```python
from build123d import *

# Parameters (mm, degrees)
SKETCH_1_W          = 113
SKETCH_1_H          = 50
SKETCH_1_R          = 1.6
SKETCH_1_R_2        = 8
SKETCH_1_R_3        = 6
EXTRUDE_1_DEPTH     = 4
SKETCH_2_R          = 1.5
SKETCH_2_R_2        = 1.6
SKETCH_2_R_3        = 2.1
CUT_EXTRUDE_1_DEPTH = 124.632519994


with BuildPart() as part:
    # ｽｹｯﾁ1 → ﾎﾞｽ - 押し出し1 (new body)
    with BuildSketch(Plane.XY):
        with Locations((56.5, 25)):
            Rectangle(SKETCH_1_W, SKETCH_1_H)
        with Locations((5, 45)):
            Circle(SKETCH_1_R, mode=Mode.SUBTRACT)
        with Locations((5, 5)):
            Circle(SKETCH_1_R, mode=Mode.SUBTRACT)
        with Locations((108, 45)):
            Circle(SKETCH_1_R, mode=Mode.SUBTRACT)
        with Locations((108, 5)):
            Circle(SKETCH_1_R, mode=Mode.SUBTRACT)
        with Locations((57.31, 25)):
            Circle(SKETCH_1_R_2, mode=Mode.SUBTRACT)
        with Locations((81.99, 25)):
            Circle(SKETCH_1_R_3, mode=Mode.SUBTRACT)
    extrude(amount=EXTRUDE_1_DEPTH)

    # ｽｹｯﾁ2 → ｶｯﾄ - 押し出し1 (cut, through all)
    with BuildSketch(Plane.XY.offset(4)):
        with Locations((90.39, 25)):
            Circle(SKETCH_2_R)
        with Locations((98.99, 46)):
            Circle(SKETCH_2_R_2)
        with Locations((98.99, 4)):
            Circle(SKETCH_2_R_2)
        with Locations((68.99, 4)):
            Circle(SKETCH_2_R_2)
        with Locations((68.99, 46)):
            Circle(SKETCH_2_R_2)
        with Locations((57.31, 39.5)):
            Circle(SKETCH_2_R_3)
        with Locations((57.31, 10.5)):
            Circle(SKETCH_2_R_3)
    extrude(amount=-CUT_EXTRUDE_1_DEPTH, mode=Mode.SUBTRACT)


solid = part.part
```
The listing builds one solid part. Answer for the finished solid, in the listing's coordinates (mm). Give positions to 0.01 mm unless a question says otherwise; leave off trailing zeros. Write each loop counter-clockwise with the first axis right and the second up, starting at its lowest first coordinate (ties: lowest second). Pieces come first, ordered by that corner, then holes. Notation, with made-up numbers: (21, 72) - (59, 72) arc R8 ccw to (59, 83) - close; hole circle Ø2 at (-8.5, 63). An arc over 180 degrees is marked (long way). Use one line per item in the form item = value. Start each with the question number.
1) Consider line 1 along Y through (x, z) = (98.99, 2.2); line 2 along Y through (x, z) = (57.31, 2.35); line 3 along X through (y, z) = (19.5, 2.4). Determine where each line is inside the solid, lowest interval first. Write a range as from..to.
2) Find section B-B on z = 1.65. Count the separate pieces of the cut face and the enclosed holes in it, plus the area to 3 significant figures.
3) The mould has two halves that part along Y. Classify faces 1 (the face through (56, 0, 2)), 2 (the face through (75.996, 25.264, 1.972)), 3 (the face through (56, 36, 0)): pulls with the +Y half, pulls with the -Y half, needs draft (parallel to the pull), parting line crosses it, or undercut.
4) Find section D-D on x = 81.99. Determine the outline of the cut face in (y, z), plus the area to 3 significant figures.
5) Find section C-C on y = 25. Determine the outline of the cut face in (x, z).
6) Find section A-A on x = 108. Determine the outline of the cut face in (y, z), plus the area to 3 significant figures.
Geometry results:
q1.line_1 = 0..2.4, 5.6..44.4, 47.6..50
q1.line_2 = 0..8.4, 12.6..17, 33..37.4, 41.6..50
q1.line_3 = 0..51.5, 63.12..79.59, 84.39..113
q2.separate_pieces = 1
q2.enclosed_holes = 13
q2.area = 5,240 mm2
q3.face_1 = pulls with the -Y half
q3.face_2 = undercut
q3.face_3 = needs draft
q4.outline = (0, 0) - (19, 0) - (19, 4) - (0, 4) - close; (31, 0) - (50, 0) - (50, 4) - (31, 4) - close
q4.area = 152 mm2
q5.outline = (0, 0) - (49.31, 0) - (49.31, 4) - (0, 4) - close; (65.31, 0) - (75.99, 0) - (75.99, 4) - (65.31, 4) - close; (87.99, 0) - (88.89, 0) - (88.89, 4) - (87.99, 4) - close; (91.89, 0) - (113, 0) - (113, 4) - (91.89, 4) - close
q6.outline = (0, 0) - (3.4, 0) - (3.4, 4) - (0, 4) - close; (6.6, 0) - (43.4, 0) - (43.4, 4) - (6.6, 4) - close; (46.6, 0) - (50, 0) - (50, 4) - (46.6, 4) - close
q6.area = 174 mm2
